Could you check a few things on this model? Use its own coordinates, in mm. A direction names the side the tool comes from. Give positions to 0.01 mm unless a question says otherwise; leave off trailing zeros. Loops run counter-clockwise (first coordinate to the right, second up) from the corner with the lowest first, then second, coordinate; pieces in that order, holes last. Notation, with made-up numbers: M 62,73.25 L 83,73.25 A31 cw 83,98.25 Z; hole C 59.25,87 d9. An arc over 180 degrees is marked long. Return JSON: item names as keys, results as strings. Group by question number.
1. Please list where these lines run through material, in increasing order: line 1 (Y direction, x = 25.5, z = 20); line 2 (X direction, y = 0, z = 34); line 3 (Z direction, x = -45, y = -12.5).
2. For pin 1 (8 mm diameter, centred on y = 14.5, z = 19.5, fed in from -X); pin 2 (19 mm diameter, centred on x = -39, z = 11.5, fed in from -Y); pin 3 (12.5 mm diameter, centred on x = 39.62, y = -0.04, fed in from +Z), each with a flat end and sliding along its axis, tell me the tip position at first contact or that it passes through.
3. If we mould it in two halves opening along Y, with no side actions, what happens to faces 5 (the flat face through (-40.8, 8.1, 25.4)), 6 (the cylindrical face through (-59.38, 0.48, 12.52)), 7 (the flat face through (-37, 16.612, 13))? For each: +Y half, -Y half, draft (parallel to the pull), parting line (faces both ways), or undercut.
4. For faces 1 (the cylindrical face through (-6.95, -16.52, 39.59)), 2 (the flat face through (-39, -14.783, 13)), 3 (the flat face through (16, 16.612, 13)), 4 (the flat face through (17, -14.783, 13)), which set-ups out of +Z, -Z, +X, -X, +Y, -Y let a thin tool reach every point of the face, with its end or its side?
5. If we section it at C-C (y = 9): Write out the boundary of the cut face in (x, z).
6. If we section it at A-A (x = 36.5): Write out the boundary of the cut face in (y, z).
7. If we section it at D-D (y = 0): Write out the boundary of the cut face in (x, z).
```python
from build123d import *

# Parameters (mm, degrees)
F0_R     = 10.927197
F2_DEPTH = 25.4
F1_R     = 18.62338
F3_DEPTH = 65.532
F4_R     = 11.856878
F5_DEPTH = 104.902


with BuildPart() as f2:
    # F0 (on Top) → F2 (new body)
    with BuildSketch(Plane.XY):
        with BuildLine():
            Line((-50.901599, -14.7828), (38.709603, -14.7828))
            ThreePointArc((38.709603, -14.7828), (54.406804, 0.9144), (38.709603, 16.6116))
            Line((38.709603, 16.6116), (-50.901599, 16.6116))
            ThreePointArc((-50.901599, 16.6116), (-66.5988, 0.9144), (-50.901599, -14.7828))
        make_face()
        with Locations((-48.463199, 0)):
            Circle(F0_R, mode=Mode.SUBTRACT)
        with BuildLine():
            ThreePointArc((11.887199, -4.7244), (7.162799, 0), (11.887199, 4.7244))
            Line((11.887199, 4.7244), (39.624002, 4.7244))
            ThreePointArc((39.624002, 4.7244), (44.370473, -0.50358), (38.709603, -4.7244))
            Line((38.709603, -4.7244), (11.887199, -4.7244))
        make_face(mode=Mode.SUBTRACT)
    extrude(amount=F2_DEPTH)

    # F1 (on Top) → F3 (join)
    with BuildSketch(Plane.XY):
        with Locations((-15.544801, 0)):
            Circle(F1_R)
    extrude(amount=F3_DEPTH)

    # F4 (on Top) → F5 (cut)
    with BuildSketch(Plane.XY):
        with Locations((-15.849601, 0)):
            Circle(F4_R)
    extrude(amount=F5_DEPTH, mode=Mode.SUBTRACT)


solid = f2.part
```
Answer:
{
 "1": {"line 1": "y = -14.78 to -4.72, 4.72 to 16.61", "line 2": "x = -34.17 to -27.71, -3.99 to 3.08", "line 3": "z = 0 to 25.4"},
 "2": {"pin 1": "stops at x = -63.33", "pin 2": "stops at y = -14.78", "pin 3": "stops at z = 25.4"},
 "3": {"face 5": "draft", "face 6": "undercut", "face 7": "+Y half"},
 "4": {"face 1": "+Z", "face 2": "+Z, -Z, -X, -Y", "face 3": "+Z, -Z, +X, +Y", "face 4": "+Z, -Z, +X, -Y"},
 "5": {"outline": "M -64.36,0 L -54.66,0 L -54.66,25.4 L -64.36,25.4 Z; M -42.27,0 L -23.57,0 L -23.57,65.53 L -31.85,65.53 L -31.85,25.4 L -42.27,25.4 Z; M -8.13,0 L 52.16,0 L 52.16,25.4 L 0.76,25.4 L 0.76,65.53 L -8.13,65.53 Z"},
 "6": {"outline": "M -14.78,0 L -4.72,0 L -4.72,25.4 L -14.78,25.4 Z; M 4.72,0 L 16.61,0 L 16.61,25.4 L 4.72,25.4 Z"},
 "7": {"outline": "M -66.57,0 L -59.39,0 L -59.39,25.4 L -66.57,25.4 Z; M -37.54,0 L -27.71,0 L -27.71,65.53 L -34.17,65.53 L -34.17,25.4 L -37.54,25.4 Z; M -3.99,0 L 7.16,0 L 7.16,25.4 L 3.08,25.4 L 3.08,65.53 L -3.99,65.53 Z; M 44.39,0 L 54.38,0 L 54.38,25.4 L 44.39,25.4 Z"}
}
